Source: three-view drawing plus pictorial views. Frame: mm from the lowest corner of the part. Give positions to 0.01 mm unless a question says otherwise; leave off trailing zeros. Write each loop counter-clockwise with the first axis right and the second up, starting at its lowest first coordinate (ties: lowest second). Pieces come first, ordered by that corner, then holes.
Q1. Draft query along Y for the marked faces 1, 2 and 3. Return one class per face: pulls with the +Y half, pulls with the -Y half, needs draft (parallel to the pull), parting line crosses it, or undercut.
Q2. Pin query (flat end, axial travel): pin 1 (5 mm diameter, centred on x = 84.43, y = 49.5, fed in from -Z); pin 2 (8 mm diameter, centred on x = 61, y = 66, fed in from -Z); pin 3 (1.5 mm diameter, centred on x = 80.5, z = 2, fed in from -Y) (1 decimal). Return the tip coordinate at first contact, or that it passes through.
Q3. Cut plane C-C on z = 1. Count the separate pieces of the cut face and the enclosed holes in it, plus the area to 3 significant figures.
Q4. Cut plane A-A on y = 47.5. Return the cut outline in (x, z).
Q5. Line query: L1, parallel to X at y = 18.5, z = 4.75; L2, parallel to X at y = 20, z = 5.25 (1 decimal); L3, parallel to Y at x = 48, z = 4.5. Output: solid intervals per line, ascending.
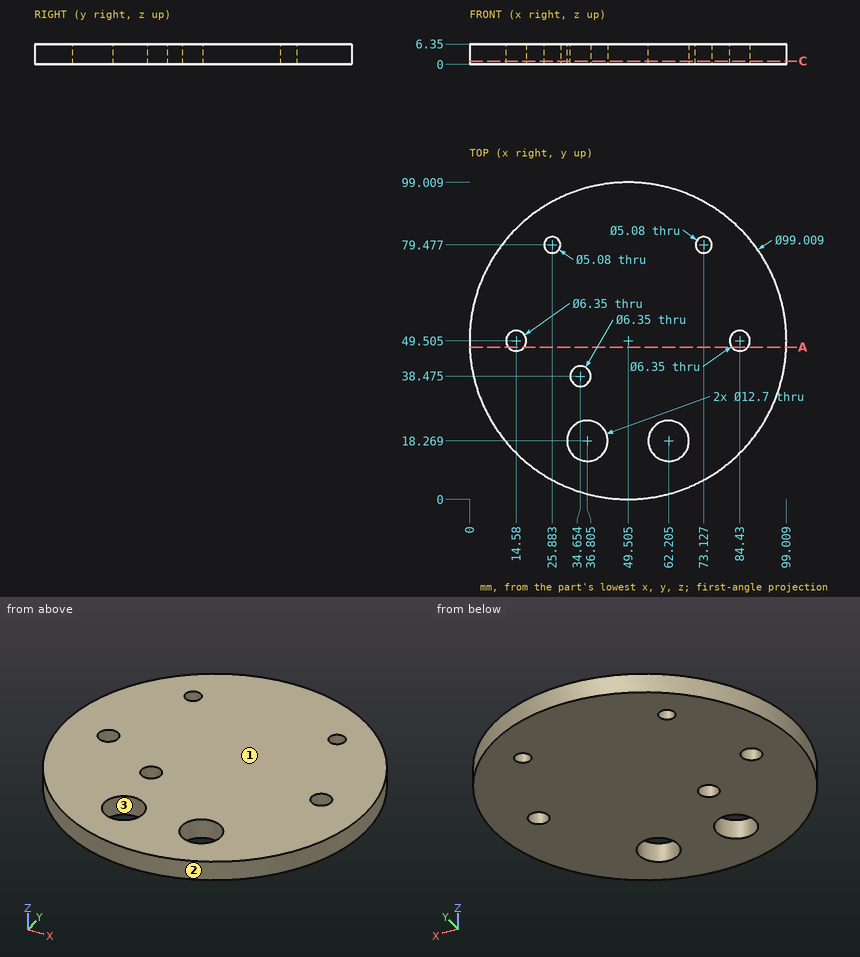
Data:
1. face 1: needs draft
1. face 2: parting line crosses it
1. face 3: undercut
2. pin 1: passes through
2. pin 2: stops at z = 0
2. pin 3: stops at y = 10.3
3. separate pieces: 1
3. enclosed holes: 7
3. area: 7,310 mm2
4. outline: (0.04, 0) - (12.12, 0) - (12.12, 6.35) - (0.04, 6.35) - close; (17.04, 0) - (81.97, 0) - (81.97, 6.35) - (17.04, 6.35) - close; (86.89, 0) - (98.97, 0) - (98.97, 6.35) - (86.89, 6.35) - close
5. L1: x = 10.91 to 30.46, 43.15 to 55.86, 68.55 to 88.1
5. L2: x = 9.8 to 30.7, 42.9 to 56.1, 68.3 to 89.3
5. L3: y = 0.02 to 98.99
